from build123d import *

# Parameters (mm, degrees)
BOSS_EXTRUDE1_DEPTH     = 15
CUT_EXTRUDE1_DEPTH      = 26
CUT_EXTRUDE1_DEPTH_BACK = 26
SKETCH2_R               = 1.05
FILLET1_R               = 2
CUT_EXTRUDE2_START      = -7
SKETCH2_3_W             = 7.5
SKETCH2_3_H             = 15
SKETCH2_3_R             = 1.05
CUT_EXTRUDE2_DEPTH      = 5
FILLET2_R               = 2
BOSS_EXTRUDE2_START     = 1
SKETCH3_R               = 1.05
BOSS_EXTRUDE2_DEPTH     = 1


with BuildPart() as part:
    # Sketch1 → Boss-Extrude1 (new body)
    with BuildSketch(Plane.XY):
        with BuildLine():
            Line((-16, 12), (-16, 0))
            Line((-16, 0), (-8.5, 0))
            ThreePointArc((-8.5, 0), (0, 8.5), (8.5, 0))
            Line((8.5, 0), (16, 0))
            Line((16, 0), (16, 12))
            Line((16, 12), (-16, 12))
        make_face()
    extrude(amount=BOSS_EXTRUDE1_DEPTH)

    # Sketch2 → Cut-Extrude1 (cut, two sides: drawn at the far end of the back side and taken through both)
    with BuildSketch(Plane.XZ.offset(-CUT_EXTRUDE1_DEPTH_BACK)):
        with Locations((-12.25, 7.5)):
            Circle(SKETCH2_R)
        with Locations(Location((12.25, 7.5, 0), (0, 0, 180))):
            Circle(SKETCH2_R)
    extrude(amount=CUT_EXTRUDE1_DEPTH + CUT_EXTRUDE1_DEPTH_BACK, mode=Mode.SUBTRACT)

    # Fillet1
    fillet1_edges = [part.edges().sort_by_distance(p)[0] for p in [
        (16, 6, 15),
        (-16, 6, 15),
        (-16, 6, 0),
        (16, 6, 0),
    ]]
    fillet(fillet1_edges, radius=FILLET1_R)

    # Sketch2<3> → Cut-Extrude2 (cut)
    # profile 1 of 2: a face of its own
    with BuildSketch(Plane.XZ.offset(CUT_EXTRUDE2_START)):
        with Locations((-12.25, 7.5)):
            Rectangle(SKETCH2_3_W, SKETCH2_3_H)
        with Locations((-12.25, 7.5)):
            Circle(SKETCH2_3_R, mode=Mode.SUBTRACT)
    # profile 2 of 2: a face of its own
    with BuildSketch(Plane.XZ.offset(CUT_EXTRUDE2_START)):
        with Locations((12.25, 7.5)):
            Rectangle(SKETCH2_3_W, SKETCH2_3_H)
        with Locations((12.25, 7.5)):
            Circle(SKETCH2_3_R, mode=Mode.SUBTRACT)
    extrude(amount=-CUT_EXTRUDE2_DEPTH, mode=Mode.SUBTRACT)

    # Fillet2
    fillet2_edges = [part.edges().sort_by_distance(p)[0] for p in [
        (-8.5, 7, 7.5),
        (-8.5, 12, 7.5),
        (8.5, 7, 7.5),
        (8.5, 12, 7.5),
    ]]
    fillet(fillet2_edges, radius=FILLET2_R)

    # Sketch3 → Boss-Extrude2 (add)
    # profile 1 of 2: a face of its own
    with BuildSketch(Plane.XZ.offset(BOSS_EXTRUDE2_START)):
        with BuildLine():
            Line((-16, 13), (-16, 2))
            ThreePointArc((-16, 2), (-15.414213562, 0.585786438), (-14, 0))
            Line((-14, 0), (-8.5, 0))
            Line((-8.5, 0), (-8.5, 15))
            Line((-8.5, 15), (-14, 15))
            ThreePointArc((-14, 15), (-15.414213562, 14.414213562), (-16, 13))
        make_face()
        with Locations((-12.25, 7.5)):
            Circle(SKETCH3_R, mode=Mode.SUBTRACT)
    # profile 2 of 2: a face of its own
    with BuildSketch(Plane.XZ.offset(BOSS_EXTRUDE2_START)):
        with BuildLine():
            Line((16, 2), (16, 13))
            ThreePointArc((16, 13), (15.414213562, 14.414213562), (14, 15))
            Line((14, 15), (8.5, 15))
            Line((8.5, 15), (8.5, 0))
            Line((8.5, 0), (14, 0))
            ThreePointArc((14, 0), (15.414213562, 0.585786438), (16, 2))
        make_face()
        with Locations((12.25, 7.5)):
            Circle(SKETCH3_R, mode=Mode.SUBTRACT)
    extrude(amount=-BOSS_EXTRUDE2_DEPTH)


solid = part.part
Here's how the part is built. I have some questions about the finished solid (model axes, mm). A direction names the side the tool comes from. Coordinates: 2 decimals unless noted, no trailing zeros. Write each loop counter-clockwise with the first axis right and the second up, starting at its lowest first coordinate (ties: lowest second). Pieces come first, ordered by that corner, then holes.
Item 1: I want a section at B-B on x = -12.25. Write out the boundary of the cut face in (y, z), and give its area (3 significant figures).
Item 2: I want a section at D-D on z = 2.75. Write out the boundary of the cut face in (x, y).
Item 3: Will these pins go through, and if not, where does the flat tip stop? pin 1 (1.9 mm diameter, centred on x = -12.25, z = 7.5, fed in from +Y); pin 2 (6 mm diameter, centred on y = 10.5, z = 10.5, fed in from -X); pin 3 (6 mm diameter, centred on x = -4, z = 10.5, fed in from -Y); pin 4 (0.8 mm diameter, centred on y = 9.5, z = 4, fed in from +X).
Item 4: If I drill on line 1 (X direction, y = -0.3, z = 7.5); line 2 (X direction, y = 2, z = 7.5); line 3 (Z direction, x = -12.25, y = -0.65), over which ranges is the centre line in solid material (lowest first)?
Item 5: If we mould it in two halves opening along X, with no side actions, what happens to faces 4 (the flat face through (8.5, -0.5, 7.6)), 5 (the flat face through (11, -1, 8)), 6 (the flat face through (-8.5, -0.5, 7.4)), 7 (the cylindrical face through (-15.4, 2.94, 14.43))? For each: +X half, -X half, draft (parallel to the pull), parting line (faces both ways), or undercut.
Item 6: I want a section at C-C on y = 2. Write out the boundary of the cut face in (x, z), and give its area (3 significant figures).
Item 7: I want a section at A-A on z = 7.5. Write out the boundary of the cut face in (x, y).
Item 8: On a 3-axis mill with a long thin cutter (end or side, diameter ignored), from which of +Z, -Z, +X, -X, +Y, -Y can I reach the whole of each face in a straight line? I mean faces 1 (the flat face through (14, 7, 8)), 2 (the flat face through (-14, 7, 8)), 3 (the flat face through (0, 10, 0)). Say none if no direction works.
Findings below:
1. outline: (-1, 0) - (7, 0) - (7, 6.45) - (-1, 6.45) - close; (-1, 8.55) - (7, 8.55) - (7, 15) - (-1, 15) - close
1. area: 103 mm2
2. outline: (-16, -1) - (-8.5, -1) - (-8.5, 0) arc R8.5 cw to (8.5, 0) - (8.5, -1) - (16, -1) - (16, 7) - (10.5, 7) arc R2 cw to (8.5, 9) - (8.5, 10) arc R2 ccw to (6.5, 12) - (-6.5, 12) arc R2 ccw to (-8.5, 10) - (-8.5, 9) arc R2 cw to (-10.5, 7) - (-16, 7) - close
3. pin 1: passes through
3. pin 2: stops at x = -9.18
3. pin 3: stops at y = 4.82
3. pin 4: stops at x = 8.5
4. line 1: x = -16 to -13.3, -11.2 to -8.5, 8.5 to 11.2, 13.3 to 16
4. line 2: x = -16 to -13.3, -11.2 to -8.26, 8.26 to 11.2, 13.3 to 16
4. line 3: z = 0 to 6.45, 8.55 to 15
5. face 4: undercut
5. face 5: draft
5. face 6: undercut
5. face 7: -X half
6. outline: (-16, 2) arc R2 ccw to (-14, 0) - (-8.26, 0) - (-8.26, 15) - (-14, 15) arc R2 ccw to (-16, 13) - close; (8.26, 0) - (14, 0) arc R2 ccw to (16, 2) - (16, 13) arc R2 ccw to (14, 15) - (8.26, 15) - close; hole circle Ø2.1 at (-12.25, 7.5); hole circle Ø2.1 at (12.25, 7.5)
6. area: 222 mm2
7. outline: (-16, -1) - (-13.3, -1) - (-13.3, 7) - (-16, 7) - close; (-11.2, -1) - (-8.5, -1) - (-8.5, 0) arc R8.5 cw to (8.5, 0) - (8.5, -1) - (11.2, -1) - (11.2, 7) - (10.5, 7) arc R2 cw to (8.5, 9) - (8.5, 10) arc R2 ccw to (6.5, 12) - (-6.5, 12) arc R2 ccw to (-8.5, 10) - (-8.5, 9) arc R2 cw to (-10.5, 7) - (-11.2, 7) - close; (13.3, -1) - (16, -1) - (16, 7) - (13.3, 7) - close
8. face 1: +Z, -Z, +X, +Y
8. face 2: +Z, -Z, -X, +Y
8. face 3: -Z, +X, -X, +Y, -Y
